```python
from build123d import *

# Parameters (mm, degrees)
SKETCH1_W               = 6
SKETCH1_H               = 5
BOSS_EXTRUDE1_DEPTH     = 33
CUT_EXTRUDE1_DEPTH      = 34.51119216
CUT_EXTRUDE1_DEPTH_BACK = 34.51119216
BOSS_EXTRUDE2_DEPTH     = 5
LPATTERN1_COUNT         = 14
LPATTERN1_PITCH         = 2
FILLET1_R               = 1


with BuildPart() as part:
    # Sketch1 → Boss-Extrude1 (new body)
    with BuildSketch(Plane(origin=(0, 0, 0), x_dir=(1, 0, 0), z_dir=(0, 1, 0))):
        Rectangle(SKETCH1_W, SKETCH1_H)
    extrude(amount=BOSS_EXTRUDE1_DEPTH)

    # Sketch2 → Cut-Extrude1 (cut, two sides: drawn at the far end of the back side and taken through both)
    with BuildSketch(Plane(origin=(0, 0, -2.5), x_dir=(-1, 0, 0), z_dir=(0, 0, -1)).offset(-CUT_EXTRUDE1_DEPTH_BACK)):
        Polygon((3, 2.5), (3, 30.7), (0.4, 28.1), (0.4, 5.1), (0.4, 0), (3, 0), align=None)
    extrude(amount=CUT_EXTRUDE1_DEPTH + CUT_EXTRUDE1_DEPTH_BACK, mode=Mode.SUBTRACT)

    # Sketch3 → Boss-Extrude2 (add)
    with BuildSketch(Plane(origin=(0, 0, -2.5), x_dir=(-1, 0, 0), z_dir=(0, 0, -1))):
        with BuildLine():
            Line((0.4, 0), (1.7, 0.75055535))
            ThreePointArc((1.7, 0.75055535), (1.8, 0.923760431), (1.7, 1.096965511))
            Line((1.7, 1.096965511), (0.4, 1.847520861))
            Line((0.4, 1.847520861), (0.4, 0))
        make_face()
    boss_extrude2 = extrude(amount=-BOSS_EXTRUDE2_DEPTH)

    # LPattern1: Boss-Extrude2 ×14
    with Locations(*[(0, i * LPATTERN1_PITCH, 0) for i in range(1, LPATTERN1_COUNT)]):
        add(boss_extrude2)

    # Fillet1
    # the kernel refuses this fillet: 1 mm, written as the material it takes off along each edge
    with BuildSketch(Plane(origin=(2, 1, -1.5), x_dir=(1, 0, 0), z_dir=(0, 0, -1))) as fillet1_piece_1_section:
        Polygon((0, 0), (FILLET1_R, 0), (FILLET1_R, FILLET1_R), (0, FILLET1_R), align=None)
    fillet1_piece_1 = extrude(amount=FILLET1_R, mode=Mode.PRIVATE)
    fillet1_piece_1 = fillet1_piece_1 - Plane(origin=(2, 1, -1.5), x_dir=(-0.7071067811865475, 0.7071067811865475, 0), z_dir=(0, 0, -1)) * Sphere(FILLET1_R, mode=Mode.PRIVATE)
    add(fillet1_piece_1, mode=Mode.SUBTRACT)
    with BuildSketch(Plane(origin=(2, 1, 1.5), x_dir=(1, 0, 0), z_dir=(0, 0, 1))) as fillet1_piece_2_section:
        Polygon((0, 0), (FILLET1_R, 0), (FILLET1_R, -FILLET1_R), (0, -FILLET1_R), align=None)
    fillet1_piece_2 = extrude(amount=FILLET1_R, mode=Mode.PRIVATE)
    fillet1_piece_2 = fillet1_piece_2 - Plane(origin=(2, 1, 1.5), x_dir=(-0.7071067811865475, 0.7071067811865475, 0), z_dir=(0, 0, 1)) * Sphere(FILLET1_R, mode=Mode.PRIVATE)
    add(fillet1_piece_2, mode=Mode.SUBTRACT)
    with BuildSketch(Plane(origin=(-2, 32, -1.5), x_dir=(-1, 0, 0), z_dir=(0, 0, -1))) as fillet1_piece_3_section:
        Polygon((0, 0), (FILLET1_R, 0), (FILLET1_R, FILLET1_R), (0, FILLET1_R), align=None)
    fillet1_piece_3 = extrude(amount=FILLET1_R, mode=Mode.PRIVATE)
    fillet1_piece_3 = fillet1_piece_3 - Plane(origin=(-2, 32, -1.5), x_dir=(0.7071067811865475, -0.7071067811865475, 0), z_dir=(0, 0, -1)) * Sphere(FILLET1_R, mode=Mode.PRIVATE)
    add(fillet1_piece_3, mode=Mode.SUBTRACT)
    with BuildSketch(Plane(origin=(-2, 32, 1.5), x_dir=(-1, 0, 0), z_dir=(0, 0, 1))) as fillet1_piece_4_section:
        Polygon((0, 0), (FILLET1_R, 0), (FILLET1_R, -FILLET1_R), (0, -FILLET1_R), align=None)
    fillet1_piece_4 = extrude(amount=FILLET1_R, mode=Mode.PRIVATE)
    fillet1_piece_4 = fillet1_piece_4 - Plane(origin=(-2, 32, 1.5), x_dir=(0.7071067811865475, -0.7071067811865475, 0), z_dir=(0, 0, 1)) * Sphere(FILLET1_R, mode=Mode.PRIVATE)
    add(fillet1_piece_4, mode=Mode.SUBTRACT)
    with BuildSketch(Plane(origin=(2, 32, 1.5), x_dir=(0, 1, 0), z_dir=(0, 0, 1))) as fillet1_piece_5_section:
        Polygon((0, 0), (FILLET1_R, 0), (FILLET1_R, -FILLET1_R), (0, -FILLET1_R), align=None)
    fillet1_piece_5 = extrude(amount=FILLET1_R, mode=Mode.PRIVATE)
    fillet1_piece_5 = fillet1_piece_5 - Plane(origin=(2, 32, 1.5), x_dir=(-0.7071067811865475, -0.7071067811865475, 0), z_dir=(0, 0, 1)) * Sphere(FILLET1_R, mode=Mode.PRIVATE)
    add(fillet1_piece_5, mode=Mode.SUBTRACT)
    with BuildSketch(Plane(origin=(2, 32, -1.5), x_dir=(0, 1, 0), z_dir=(0, 0, -1))) as fillet1_piece_6_section:
        Polygon((0, 0), (FILLET1_R, 0), (FILLET1_R, FILLET1_R), (0, FILLET1_R), align=None)
    fillet1_piece_6 = extrude(amount=FILLET1_R, mode=Mode.PRIVATE)
    fillet1_piece_6 = fillet1_piece_6 - Plane(origin=(2, 32, -1.5), x_dir=(-0.7071067811865475, -0.7071067811865475, 0), z_dir=(0, 0, -1)) * Sphere(FILLET1_R, mode=Mode.PRIVATE)
    add(fillet1_piece_6, mode=Mode.SUBTRACT)
    with BuildSketch(Plane(origin=(2, 0, -2.5), x_dir=(0, 0, 1), z_dir=(-1, 0, 0))) as fillet1_piece_7:
        with BuildLine():
            CenterArc((FILLET1_R, FILLET1_R), FILLET1_R, 180, 90)
            Line((0, FILLET1_R), (0, 0))
            Line((0, 0), (FILLET1_R, 0))
        make_face()
    extrude(amount=4.9, mode=Mode.SUBTRACT)
    with BuildSketch(Plane(origin=(-2.9, 0, 2.5), x_dir=(0, 1, 0), z_dir=(1, 0, 0))) as fillet1_piece_8:
        with BuildLine():
            CenterArc((FILLET1_R, -FILLET1_R), FILLET1_R, 90, 90)
            Line((0, -FILLET1_R), (0, 0))
            Line((0, 0), (FILLET1_R, 0))
        make_face()
    extrude(amount=4.9, mode=Mode.SUBTRACT)
    with BuildSketch(Plane(origin=(-3, 33, -1.5), x_dir=(0, -1, 0), z_dir=(0, 0, 1))) as fillet1_piece_9:
        with BuildLine():
            CenterArc((FILLET1_R, FILLET1_R), FILLET1_R, 180, 90)
            Line((0, FILLET1_R), (0, 0))
            Line((0, 0), (FILLET1_R, 0))
        make_face()
    extrude(amount=3, mode=Mode.SUBTRACT)
    with BuildSketch(Plane(origin=(-3, 28.2, 2.5), x_dir=(1, 0, 0), z_dir=(0, 1, 0)), Plane(origin=(-3, 28.2, -2.5), x_dir=(0, 0, 1), z_dir=(0, 1, 0))) as fillet1_piece_10:
        with BuildLine():
            CenterArc((FILLET1_R, FILLET1_R), FILLET1_R, 180, 90)
            Line((0, FILLET1_R), (0, 0))
            Line((0, 0), (FILLET1_R, 0))
        make_face()
    extrude(amount=3.8, mode=Mode.SUBTRACT)
    with BuildSketch(Plane(origin=(-3, 30.7, 3.535533906), x_dir=(0.7071067811865411, -0.7071067811865539, 0), z_dir=(0, 0, -1))) as fillet1_piece_11:
        with BuildLine():
            CenterArc((FILLET1_R * 0.414213562373, -FILLET1_R), FILLET1_R, 90, 45)
            Line((-FILLET1_R * 0.292893218813, -FILLET1_R * 0.292893218813), (0, 0))
            Line((0, 0), (FILLET1_R * 0.414213562373, 0))
        make_face()
    extrude(amount=7.071067812, mode=Mode.SUBTRACT)
    with BuildSketch(Plane(origin=(3, 1, 2.5), x_dir=(-1, 0, 0), z_dir=(0, 1, 0)), Plane(origin=(3, 1, -2.5), x_dir=(0, 0, 1), z_dir=(0, 1, 0))) as fillet1_piece_12:
        with BuildLine():
            CenterArc((FILLET1_R, -FILLET1_R), FILLET1_R, 90, 90)
            Line((0, -FILLET1_R), (0, 0))
            Line((0, 0), (FILLET1_R, 0))
        make_face()
    extrude(amount=31, mode=Mode.SUBTRACT)
    with BuildSketch(Plane(origin=(3, 33, 1.5), x_dir=(-1, 0, 0), z_dir=(0, 0, -1)), Plane(origin=(3, 0, 1.5), x_dir=(0, 1, 0), z_dir=(0, 0, -1))) as fillet1_piece_13:
        with BuildLine():
            CenterArc((FILLET1_R, -FILLET1_R), FILLET1_R, 90, 90)
            Line((0, -FILLET1_R), (0, 0))
            Line((0, 0), (FILLET1_R, 0))
        make_face()
    extrude(amount=3, mode=Mode.SUBTRACT)
    with BuildSketch(Plane(origin=(-2, 33, 2.5), x_dir=(0, -1, 0), z_dir=(1, 0, 0))) as fillet1_piece_14:
        with BuildLine():
            CenterArc((FILLET1_R, FILLET1_R), FILLET1_R, 180, 90)
            Line((0, FILLET1_R), (0, 0))
            Line((0, 0), (FILLET1_R, 0))
        make_face()
    extrude(amount=4, mode=Mode.SUBTRACT)
    with BuildSketch(Plane(origin=(2, 33, -2.5), x_dir=(0, 0, 1), z_dir=(-1, 0, 0))) as fillet1_piece_15:
        with BuildLine():
            CenterArc((FILLET1_R, -FILLET1_R), FILLET1_R, 90, 90)
            Line((0, -FILLET1_R), (0, 0))
            Line((0, 0), (FILLET1_R, 0))
        make_face()
    extrude(amount=4, mode=Mode.SUBTRACT)
    with BuildSketch(Plane(origin=(-0.4, 0, -3.169872981), x_dir=(1, 0, 0), z_dir=(0, 0, 1))) as fillet1_piece_16:
        with BuildLine():
            CenterArc((FILLET1_R * 0.267949192431, FILLET1_R), FILLET1_R, 240, 30)
            Line((-FILLET1_R * 0.232050807569, FILLET1_R * 0.133974596216), (0, 0))
            Line((0, 0), (FILLET1_R * 0.267949192431, 0))
        make_face()
    extrude(amount=6.339745962, mode=Mode.SUBTRACT)


solid = part.part
```
Source: CAD feature listing. Evaluate the final solid. Frame: model axes, mm. A direction names the side the tool comes from. Coordinates: 2 decimals unless noted, no trailing zeros. Answer as a JSON object with one key per item and string values.
1. Cut plane A-A on x = -1. State how many separate pieces and enclosed holes the cut face has, plus the area to 3 significant figures.
Evaluation:
{"separate pieces": "15", "enclosed holes": "0", "area": "102 mm^2"}
2. Contact query for flat-ended pins moving along their axis: P1, Ø1, axis at y = 25, z = -0.5, coming from the -X side; P2, Ø2, axis at x = 0, z = 2, coming from the -Y side. Output: stop coordinate, or through.
Evaluation:
{"P1": "x = -1.8", "P2": "y = 0"}
3. Ray query, L1, parallel to X at y = 31.5, z = -1.55; L2, parallel to Z at x = 2.5, y = 3; L3, parallel to X at y = 28, z = -1.15. Return the intervals inside material, ascending.
Evaluation:
{"L1": "-3 to 3", "L2": "-2.37 to 2.37", "L3": "-0.4 to 3"}
4. Draft query along Y for faces 3 (the cylindrical face through (0.494, 0.301, 2.215)), 4 (the cylindrical face through (2.715, 16.283, -2.199)), 5 (the flat face through (-1.04, 2.37, -0.04)), 6 (the cylindrical face through (-2.699, 32.715, -0.021)). Return one class per face: released by +Y, released by -Y, zero draft, split by the parting line, or undercut.
Evaluation:
{"face 3": "released by -Y", "face 4": "zero draft", "face 5": "undercut", "face 6": "released by +Y"}
5. Access query for faces 1 (the flat face through (-1.059, 19.467, -0.035)), 2 (the cylindrical face through (2.715, 0.301, 0.021)). Directions: +Z, -Z, +X, -X, +Y, -Y. A direction counts if a zero-diameter tool reaches every point of the face in a straight line with its end or side. Return the directions, or none.
Evaluation:
{"face 1": "+Z, -Z, -X", "face 2": "+Z, -Z, +X, -Y"}
